Part print with two shaded views. Sizes in mm from the minimum x, y, z corner. A direction names the side the tool comes from. Give positions to 0.01 mm unless a question says otherwise; leave off trailing zeros. Write each loop counter-clockwise with the first axis right and the second up, starting at its lowest first coordinate (ties: lowest second). Pieces come first, ordered by that corner, then holes. Notation, with made-up numbers: M -24.5,86.5 L -9.5,86.5 A14 cw -9.5,113.5 Z; hole C 7.25,26.25 d7. An arc over 180 degrees is marked long. Return JSON: item names as keys, results as strings. Group by question number.
Q1. Band-saw the part on B-B, the plane x = 33.5. Give the cut face in (y, z), then the cut area to 3 significant figures.
Q2. Pull direction Z, two halves, no side cores. Call the marked faces 4, 5 and 6: +Z half, -Z half, draft (parallel to the pull), parting line (faces both ways), or undercut.
Q3. Tool access for the marked faces 1, 2 and 3: list every direction of +Z, -Z, +X, -X, +Y, -Y with a clear straight run to the whole face (end or side of a thin tool).
Q4. Band-saw the part on C-C, the plane z = 57. Give the cut face in (x, y), then the cut area to 4 significant figures.
Q5. Flat gauge pins, fed straight in: pin 1 Ø20 at (x, z) = (34.5, 57.5) entering from +Y; pin 2 Ø25 at (x, y) = (18, 52) entering from +Z; pin 3 Ø12.5 at (y, z) = (51, 51.5) entering from +X. Where does each tip first touch, or does it go through?
Q6. Wall check: probe 1 along Z at (x, y) = (19.5, 24); probe 2 along Z at (x, y) = (8, 3.5); probe 3 along Y at (x, z) = (28.5, 8.5). Give the ranges that are in metal, low to high.
Q7. Band-saw the part on D-D, the plane y = 44. Give the cut face in (x, z), then the cut area to 3 significant figures.
Q8. Band-saw the part on A-A, the plane y = 57.5. Give the cut face in (x, z).
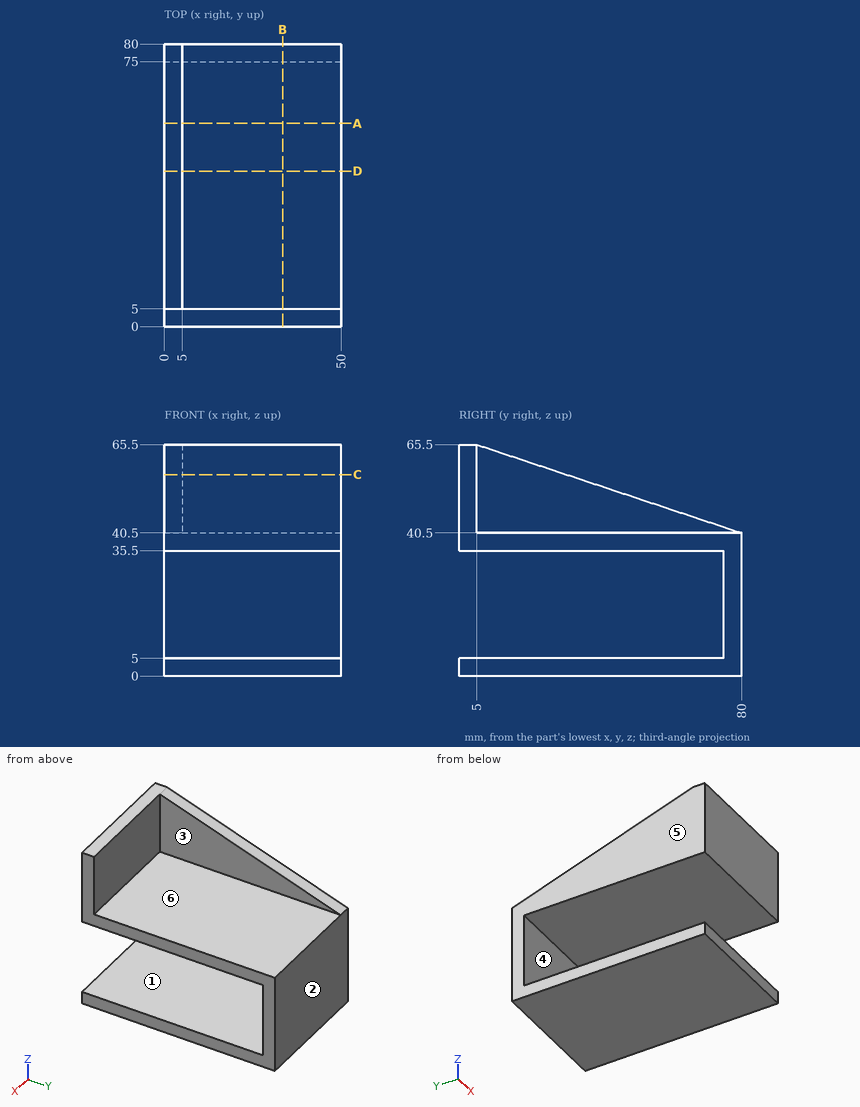
From the geometry:
{
 "1": {"outline": "M 0,0 L 80,0 L 80,40.5 L 5,40.5 L 5,65.5 L 0,65.5 L 0,35.5 L 75,35.5 L 75,5 L 0,5 Z", "area": "1,080 mm^2"},
 "2": {"face 4": "undercut", "face 5": "draft", "face 6": "+Z half"},
 "3": {"face 1": "+X, -X, -Y", "face 2": "+Z, -Z, +X, -X, +Y", "face 3": "+Z, +X, +Y"},
 "4": {"outline": "M 0,0 L 50,0 L 50,5 L 5,5 L 5,30.5 L 0,30.5 Z", "area": "377.5 mm^2"},
 "5": {"pin 1": "stops at y = 5", "pin 2": "stops at z = 40.5", "pin 3": "stops at x = 5"},
 "6": {"probe 1": "z = 0 to 5, 35.5 to 40.5", "probe 2": "z = 0 to 5, 35.5 to 65.5", "probe 3": "y = 75 to 80"},
 "7": {"outline": "M 0,0 L 50,0 L 50,5 L 0,5 Z; M 0,35.5 L 50,35.5 L 50,40.5 L 5,40.5 L 5,52.5 L 0,52.5 Z", "area": "560 mm^2"},
 "8": {"outline": "M 0,0 L 50,0 L 50,5 L 0,5 Z; M 0,35.5 L 50,35.5 L 50,40.5 L 5,40.5 L 5,48 L 0,48 Z"}
}
